from build123d import *

# Parameters (mm, degrees)
F1_DEPTH = 100


with BuildPart() as f1:
    # F0 (on Top) → F1 (new body)
    with BuildSketch(Plane.XY):
        with BuildLine():
            ThreePointArc((0, 35.794553), (-45, 57.5), (-90, 35.794553))
            ThreePointArc((-90, 35.794553), (-192.5, 0), (-90, -35.794553))
            ThreePointArc((-90, -35.794553), (-45, -57.5), (0, -35.794553))
            ThreePointArc((0, -35.794553), (45, -57.5), (90, -35.794553))
            ThreePointArc((90, -35.794553), (192.5, 0), (90, 35.794553))
            ThreePointArc((90, 35.794553), (45, 57.5), (0, 35.794553))
        make_face()
        with BuildLine():
            ThreePointArc((-90, -15.206906), (-182.5, 0), (-90, 15.206906))
            ThreePointArc((-90, 15.206906), (-45, 47.5), (0, 15.206906))
            ThreePointArc((0, 15.206906), (45, 47.5), (90, 15.206906))
            ThreePointArc((90, 15.206906), (182.5, 0), (90, -15.206906))
            ThreePointArc((90, -15.206906), (45, -47.5), (0, -15.206906))
            ThreePointArc((0, -15.206906), (-45, -47.5), (-90, -15.206906))
        make_face(mode=Mode.SUBTRACT)
    extrude(amount=-F1_DEPTH)


solid = f1.part
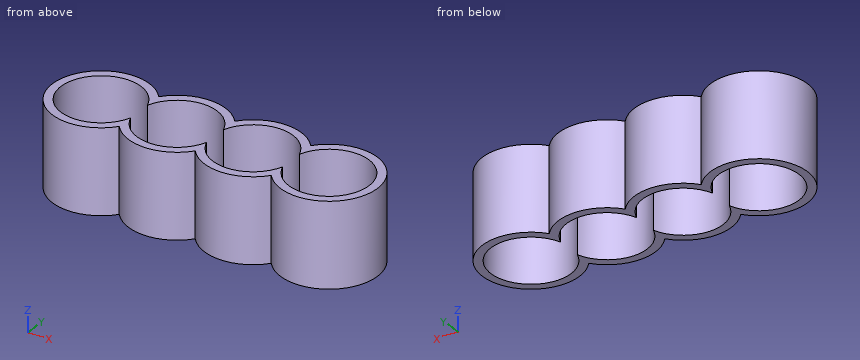
Model file for the job. Use its own axes, mm. Round coordinates to 2 decimals unless told otherwise and drop trailing zeros. Loops run counter-clockwise (first coordinate to the right, second up) from the corner with the lowest first, then second, coordinate; pieces in that order, holes last. Notation, with made-up numbers: M 71,49.25 L 97,49.25 A27 cw 97,70.25 Z; hole C -34.5,3 d1. An arc over 180 degrees is marked long. One line per question, with ' | ' between items.
1) Band-saw the part on B-B (z = -74.5). Give the cut face in (x, y), then the cut area to 3 significant figures.
Solved:
outline: M -90,-35.79 A57.5 ccw 0,-35.79 A57.5 ccw 90,-35.79 A57.5 ccw long 90,35.79 A57.5 ccw 0,35.79 A57.5 ccw -90,35.79 A57.5 ccw long Z; hole M -90,-15.21 A47.5 ccw 0,-15.21 A47.5 ccw 90,-15.21 A47.5 ccw long 90,15.21 A47.5 ccw 0,15.21 A47.5 ccw -90,15.21 A47.5 ccw long Z | area: 9,840 mm²
2) Drill centre lines: line 1 along Y through (x, z) = (-43, -56); line 2 along X through (y, z) = (26, -61.5); line 3 along X through (y, z) = (27.5, -89.5). Where is each one in solid material? Low to high.
Solved:
line 1: y = -57.47 to -47.46, 47.46 to 57.47 | line 2: x = -186.29 to -174.75, -95.25 to -84.75, -5.25 to 5.25, 84.75 to 95.25, 174.75 to 186.29 | line 3: x = -185.5 to -173.73, -96.27 to -83.73, -6.27 to 6.27, 83.73 to 96.27, 173.73 to 185.5
3) Band-saw the part on C-C (y = 0). Give the cut face in (x, z), then the cut area to 3 significant figures.
Solved:
outline: M -192.5,-100 L -182.5,-100 L -182.5,0 L -192.5,0 Z; M 182.5,-100 L 192.5,-100 L 192.5,0 L 182.5,0 Z | area: 2,000 mm²
4) Band-saw the part on A-A (x = -135). Give the cut face in (y, z).
Solved:
outline: M -57.5,-100 L -47.5,-100 L -47.5,0 L -57.5,0 Z; M 47.5,-100 L 57.5,-100 L 57.5,0 L 47.5,0 Z
5) Band-saw the part on D-D (y = -19). Give the cut face in (x, z).
Solved:
outline: M -189.27,-100 L -178.53,-100 L -178.53,0 L -189.27,0 Z; M -91.47,-100 L -88.53,-100 L -88.53,0 L -91.47,0 Z; M -1.47,-100 L 1.47,-100 L 1.47,0 L -1.47,0 Z; M 88.53,-100 L 91.47,-100 L 91.47,0 L 88.53,0 Z; M 178.53,-100 L 189.27,-100 L 189.27,0 L 178.53,0 Z
6) Flat gauge pins, fed straight in: pin 1 (8 mm diameter, centred on y = 45.5, z = -29, fed in from +X); pin 2 (1 mm diameter, centred on x = -92, z = -86.5, fed in from -Y); pin 3 (12 mm diameter, centred on x = -93.5, y = -14, fed in from -Z); pin 4 (4 mm diameter, centred on x = 65, z = -72.5, fed in from +Y). Where does each tip first touch, or does it go through?
Solved:
pin 1: stops at x = 174.8 | pin 2: stops at y = -38.73 | pin 3: stops at z = -100 | pin 4: stops at y = 54.61
